```python
from build123d import *

# Parameters (mm, degrees)
F1_DEPTH    = 5
F2_R        = 2.75
F3_DEPTH    = 58.2
F4_R        = 2
F5_DEPTH    = 25
F1_FACE_R   = 2.75
F1_FACE_R_2 = 2
F6_DEPTH    = 5


with BuildPart() as f1:
    # F0 (on Top) → F1 (new body)
    with BuildSketch(Plane.XY):
        Polygon((31, 0), (0, 0), (-31, 0), (-31, 10), (-45, 10), (-45, -30), (45, -30), (45, 10), (31, 10), align=None)
    extrude(amount=F1_DEPTH)

    # F2 (on Top) → F3 (cut)
    with BuildSketch(Plane.XY):
        with Locations((-34.98394, -19.975932)):
            Circle(F2_R)
        with Locations((-35.002254, 0)):
            Circle(F2_R)
        with Locations((34.966677, 0)):
            Circle(F2_R)
        with Locations((34.966677, -19.899994)):
            Circle(F2_R)
    extrude(amount=F3_DEPTH, mode=Mode.SUBTRACT)

    # F4 (on face) → F5 (cut)
    with BuildSketch(Plane.XY.offset(5)):
        with Locations((-14.981076, -14.93126)):
            Circle(F4_R)
        with Locations((15.037959, -14.93126)):
            Circle(F4_R)
    extrude(amount=-F5_DEPTH, mode=Mode.SUBTRACT)

    # F1_face (on face) → F6 (join)
    with BuildSketch(Plane(origin=(0.000435, -13.224629, 5), x_dir=(1, 0, 0), z_dir=(0, 0, 1))):
        Polygon((30.999565, 13.224629), (-31.000435, 13.224629), (-31.000435, 23.224629), (-45.000435, 23.224629), (-45.000435, -16.775371), (44.999565, -16.775371), (44.999565, 23.224629), (30.999565, 23.224629), align=None)
        with Locations((-34.984376, -6.751303)):
            Circle(F1_FACE_R, mode=Mode.SUBTRACT)
        with Locations((-14.981511, -1.706631)):
            Circle(F1_FACE_R_2, mode=Mode.SUBTRACT)
        with Locations((34.966242, -6.675365)):
            Circle(F1_FACE_R, mode=Mode.SUBTRACT)
        with Locations((15.037524, -1.706631)):
            Circle(F1_FACE_R_2, mode=Mode.SUBTRACT)
        with Locations((-35.002689, 13.224629)):
            Circle(F1_FACE_R, mode=Mode.SUBTRACT)
        with Locations((34.966242, 13.224629)):
            Circle(F1_FACE_R, mode=Mode.SUBTRACT)
    extrude(amount=F6_DEPTH)


solid = f1.part
```
Geometry check sheet. Reference: the model listing, model coordinates, mm. A direction names the side the tool comes from. Round coordinates to 2 decimals unless told otherwise and drop trailing zeros. Loops run counter-clockwise (first coordinate to the right, second up) from the corner with the lowest first, then second, coordinate; pieces in that order, holes last. Notation, with made-up numbers: M 15,-28 L 59,-28 A10 ccw 59,-12 Z; hole C 45,38.25 d9. An arc over 180 degrees is marked long. Return JSON: item names as keys, results as strings. Group by question number.
(1) Section check A-A, the plane y = -19. Give the number of separate pieces and of enclosed holes in the cut face, and give its area (3 significant figures).
(2) Section check C-C, the plane x = -1.5. Enter the section's corners in (y, z), and give its area (3 significant figures).
(3) Go/stop test with flat-tipped pins: pin 1 (3.5 mm diameter, centred on x = 15.04, y = -14.93, fed in from -Z); pin 2 (9 mm diameter, centred on x = 34.97, y = -19.9, fed in from +Z); pin 3 (3 mm diameter, centred on x = -23, z = 3, fed in from +Y). Record where each tip stops, or that it passes through.
(4) Section check B-B, the plane z = 2. Enter the section's corners in (x, y).
(5) Mould release check, pull along Y, two halves, no side actions. Record for faces 1 (the face through (-1, -30, 5)), 2 (the face through (-38, 10, 5)), 3 (the face through (-37.75, 0.12, 4.93)), 4 (the face through (31, 5, 5)): pulls with the +Y half, pulls with the -Y half, needs draft (parallel to the pull), parting line crosses it, or undercut.
(6) Set-up check for faces 5 (the face through (0, 0, 5)), 6 (the face through (-1, -14, 10)): record each of +Z, -Z, +X, -X, +Y, -Y from which the full face is reachable in a straight line by a thin tool's end or side.
(7) Scan lines: line 1 along X through (y, z) = (-2, 7); line 2 along X through (y, z) = (3.5, 4.75); line 3 along X through (y, z) = (-22, 4.5). Record each from-to range of solid material in increasing order. Write a range as [from, to].
Data:
{
 "1": {"separate pieces": "3", "enclosed holes": "0", "area": "797 mm²"},
 "2": {"outline": "M -30,0 L 0,0 L 0,10 L -30,10 Z", "area": "300 mm²"},
 "3": {"pin 1": "through", "pin 2": "z = 10", "pin 3": "y = 0"},
 "4": {"outline": "M -45,-30 L 45,-30 L 45,10 L 31,10 L 31,0 L -31,0 L -31,10 L -45,10 Z; hole C -35,0 d5.5; hole C -34.98,-19.98 d5.5; hole C -14.98,-14.93 d4; hole C 15.04,-14.93 d4; hole C 34.97,-19.9 d5.5; hole C 34.97,0 d5.5"},
 "5": {"face 1": "pulls with the -Y half", "face 2": "pulls with the +Y half", "face 3": "undercut", "face 4": "needs draft"},
 "6": {"face 5": "+Z, -Z, +Y", "face 6": "+Z, +X, -X, +Y, -Y"},
 "7": {"line 1": "[-45, -36.89], [-33.11, 33.08], [36.85, 45]", "line 2": "[-45, -31], [31, 45]", "line 3": "[-45, -36.85], [-33.12, 33.19], [36.74, 45]"}
}
